Geometry: see drawing. Coordinates: mm, zero at the bounding-box minimum. Give positions to 0.01 mm unless a question says otherwise; leave off trailing zeros. Write each loop counter-clockwise with the first axis right and the second up, starting at its lowest first coordinate (ties: lowest second). Pieces come first, ordered by that corner, then holes. Notation, with made-up numbers: M -40,-31 L 14,-31 A9 cw 14,-20 Z; hole C 51,8 d1. An arc over 180 degrees is marked long. Use CSV: the item, a comma, the result in double quotes. Start each with the question number.
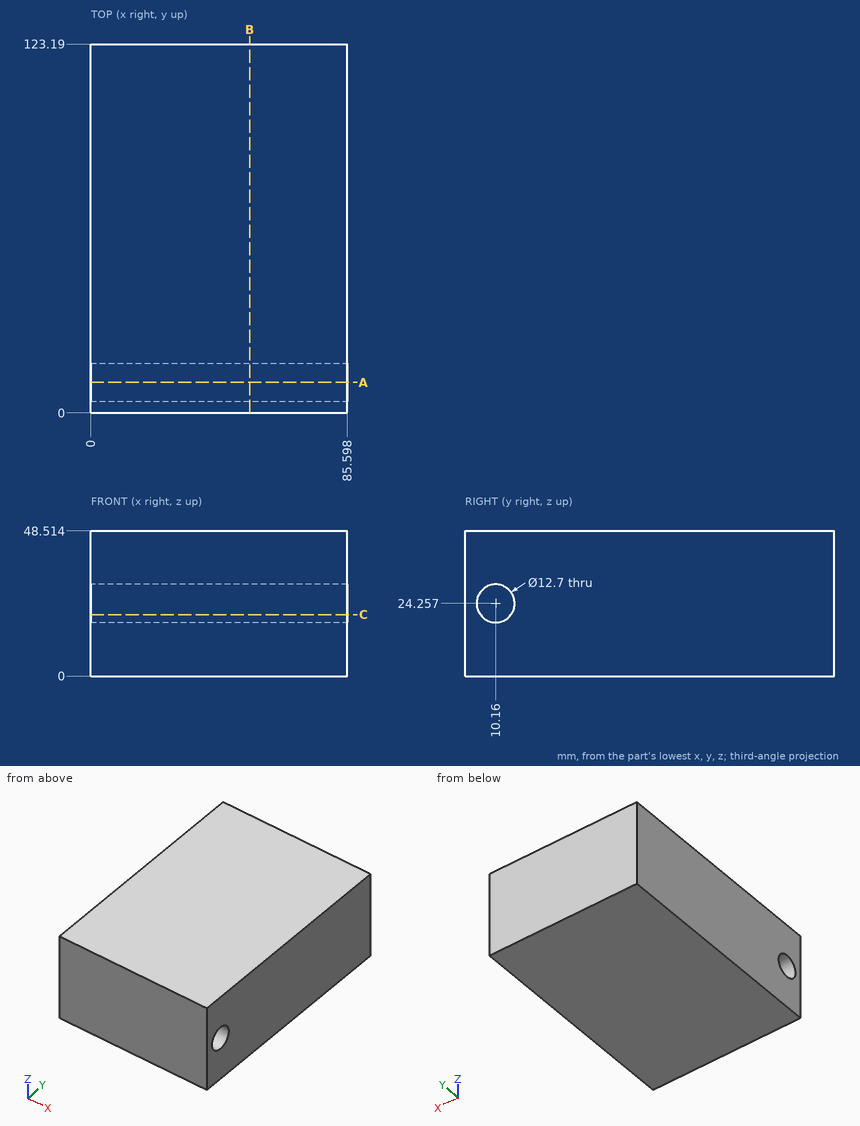
1. Section B-B on x = 53. Return loops of the section in (y, z).
2. Section C-C on z = 20.5. Return loops of the section in (x, y).
3. First-contact query: pin 1 (5 mm diameter, centred on x = 37, y = 74.5, fed in from -Z). Flat tip, straight axial feed; report the tip coordinate or a pass-through.
4. Line query: probe 1 along Z at (x, y) = (21, 10); probe 2 along Y at (x, z) = (48, 27); probe 3 along Z at (x, y) = (17, 15). Output: solid intervals per line, ascending.
5. Section A-A on y = 10.16. Return loops of the section in (x, z), then the cut area to 3 significant figures.
Resolved:
1,outline,"M 0,0 L 123.19,0 L 123.19,48.51 L 0,48.51 Z; hole C 10.16,24.26 d12.7"
2,outline,"M 0,0 L 85.6,0 L 85.6,5.04 L 0,5.04 Z; M 0,15.28 L 85.6,15.28 L 85.6,123.19 L 0,123.19 Z"
3,pin 1,"stops at z = 0"
4,probe 1,"z = 0 to 17.91, 30.6 to 48.51"
4,probe 2,"y = 0 to 4.43, 15.89 to 123.19"
4,probe 3,"z = 0 to 20.15, 28.37 to 48.51"
5,outline,"M 0,0 L 85.6,0 L 85.6,17.91 L 0,17.91 Z; M 0,30.61 L 85.6,30.61 L 85.6,48.51 L 0,48.51 Z"
5,area,"3,070 mm2"
